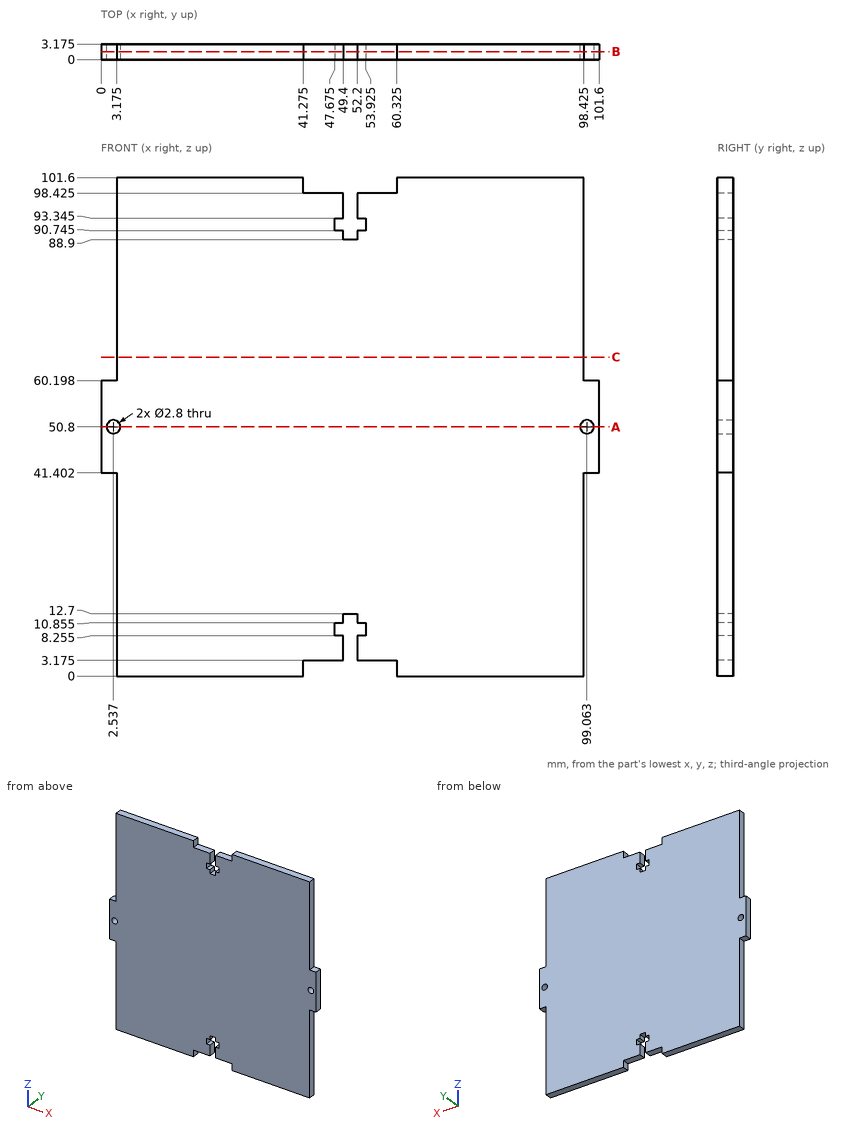
For this review, use the dimensioned drawing (mm, ordinates from the lowest corner) and the shaded views. Give positions to 0.01 mm unless a question says otherwise; leave off trailing zeros. Order: outer loops, then holes, each group sorted by start corner. A loop starts at its lowest first (then second) coordinate and runs counter-clockwise, first axis right, second up.
1. Add section C-C, the plane z = 65. State the section outline as (x, y) points (3 decimals), then the cut area to 3 significant figures.
Solution:
outline: (3.175, 0) - (98.425, 0) - (98.425, 3.175) - (3.175, 3.175) - close
area: 302 mm2
2. For pin 1 Ø1 at (y, z) = (1.5, 101) entering from -X (3 decimals); pin 2 Ø0.9 at (y, z) = (1.5, 90) entering from +X (3 decimals); pin 3 Ø0.9 at (x, y) = (53, 2) entering from +Z (3 decimals), all flat-tipped, find the tip position at first contact; note any pin that passes through.
Solution:
pin 1: stops at x = 3.175
pin 2: stops at x = 98.425
pin 3: stops at z = 98.425
3. To check wall thickness, follow L1, parallel to Z at x = 48, y = 1.5 (3 decimals); L2, parallel to X at y = 0.8, z = 11 (3 decimals); L3, parallel to Z at x = 43.5, y = 3.05 (3 decimals). State the ranges of each line that lie inside material, in increasing order.
Solution:
L1: z = 3.175 to 8.255, 10.855 to 90.745, 93.345 to 98.425
L2: x = 3.175 to 49.4, 52.2 to 98.425
L3: z = 3.175 to 98.425
4. Add section A-A, the plane z = 50.8. State the section outline as (x, y) points (3 decimals), then the cut area to 3 significant figures.
Solution:
outline: (0, 0) - (1.137, 0) - (1.137, 3.175) - (0, 3.175) - close; (3.937, 0) - (97.663, 0) - (97.663, 3.175) - (3.937, 3.175) - close; (100.463, 0) - (101.6, 0) - (101.6, 3.175) - (100.463, 3.175) - close
area: 305 mm2
5. Add section B-B, the plane y = 1.6. State how many separate pieces and enclosed holes the cut face has, then the cut area to 3 significant figures.
Solution:
separate pieces: 1
enclosed holes: 2
area: 9,590 mm2
